Autodesk Inventor part; units mm, degrees
ref_plane "YZ Plane" through (0, 0, 0) normal (1, 0, 0) x (0, 1, 0)
ref_plane "XZ Plane" through (0, 0, 0) normal (0, 1, 0) x (-1, 0, 0)
ref_plane "XY Plane" through (0, 0, 0) normal (0, 0, 1) x (1, 0, 0)
sketch "Sketch1" plane through (0, 0, 0) normal (0, 1, 0) x (-1, 0, 0)
  line L0 (-60, 0) -> (-940, 0)
  line L1 (-891.5776, 120) -> (-60, 120)
  arc A0 (-60, 0) -> (-60, 120) centre (-60, 60) ccw
  line L2 (-60, 0) -> (-90, 0)
  arc A1 (-1909.8969, 691.9019) -> (-1970.1031, 588.0981) centre (-1940, 640) ccw
  line L3 (-1909.8969, 691.9019) -> (-951.7838, 136.1963)
  line L4 (-1970.1031, 588.0981) -> (-970.1031, 8.0981)
  arc A2 (-951.7838, 136.1963) -> (-891.5776, 120) centre (-891.5776, 240) ccw
  arc A3 (-970.1031, 8.0981) -> (-940, 0) centre (-940, 60) ccw
  line L5 (-60, 0) -> (-110, 0)
  line L6 (-110, 0) -> (-110, -100)
  line L7 (-110, -100) -> (-60, -100)
  line L8 (-60, -100) -> (-60, 0)
  line L9 (-940, 0) -> (-890, 0)
  line L10 (-890, 0) -> (-890, -100)
  line L11 (-890, -100) -> (-940, -100)
  line L12 (-940, -100) -> (-940, 0)
  line L13 (-1920.1031, 559.0981) -> (-1920.1031, -199.9999)
  line L14 (-1920.1031, -199.9999) -> (-1970.1031, -199.9999)
  line L15 (-1970.1031, -199.9999) -> (-1970.1031, 588.0981)
  point P0 (0, 0)
  dimension "d9" = 120
  dimension "d10" = 50
  dimension "d11" = 100
  dimension "d12" = 50
  dimension "d13" = 100
  dimension "d16" = 50
extrude "Extrusion1" add sketch "Sketch1" against normal blind 50 contours L8 L7 L6 L0 | L10 L11 L12 L0 | L4 L13 L14 L15
extrude "Extrusion2" add sketch "Sketch1" against normal blind 450 contours L0 A3 L4 A1 L3 A2 L1 A0
extrude "Extrusion3" add sketch "Sketch1" along normal blind 50 contours L0 A3 L4 A1 L3 A2 L1 A0
sketch "Sketch2" plane through (940, -450, 0) normal (0, 0, -1) x (-1, 0, 0)
  line L0 (880, 400) -> (880, 0)
  line L1 (880, 50) -> (830, 50)
  line L2 (830, 50) -> (830, 100)
  line L3 (830, 100) -> (880, 100)
  line L4 (880, 100) -> (880, 50)
  line L5 (0, 400) -> (0, 0)
  line L6 (0, 50) -> (50, 50)
  line L7 (50, 50) -> (50, 100)
  line L8 (50, 100) -> (0, 100)
  line L9 (0, 100) -> (0, 50)
  line L10 (-1030.1031, 50) -> (-980.1031, 50)
  line L11 (-980.1031, 50) -> (-980.1031, 100)
  line L12 (-980.1031, 100) -> (-1030.1031, 100)
  line L13 (-1030.1031, 100) -> (-1030.1031, 50)
  point P0 (940, 450)
  dimension "d24" = 50
  dimension "d25" = 50
  dimension "d26" = 50
  dimension "d27" = 50
  dimension "d28" = 50
  dimension "d29" = 50
extrude "Extrusion4" add sketch "Sketch2" along normal blind 100 contours L0 L1 L2 L3 | L8 L7 L6 L5
extrude "Extrusion5" add sketch "Sketch2" along normal blind 200 contours L13 L12 L11 L10
extrude "Extrusion6" add sketch "Sketch2" against normal blind 600 contours L13 L12 L11 L10
properties part number "FirstConveyor"
The model under review builds one solid part; all positions refer to its coordinate system, in mm. A direction names the side the tool comes from. Round coordinates to 2 decimals unless told otherwise and drop trailing zeros. Order: outer loops, then holes, each group sorted by start corner. A loop starts at its lowest first (then second) coordinate and runs counter-clockwise, first axis right, second up.
Item 1: Draft analysis for pull direction X (two halves, no side actions). For faces 4 (the flat face through (494, -204, 0)), 5 (the flat face through (1970.103, -25, 189)), 6 (the flat face through (85, -350, -49)), state which applies: released by +X, released by -X, zero draft, split by the parting line, or undercut.
Working result:
face 4: undercut
face 5: released by +X
face 6: zero draft
Item 2: Add section C-C, the plane x = 1940. State the section outline as (y, z) points.
Working result:
outline: (-450, 570.64) - (-400, 570.64) - (-400, -200) - (-350, -200) - (-350, 570.64) - (-50, 570.64) - (-50, -200) - (0, -200) - (0, 570.64) - (50, 570.64) - (50, 700) - (-450, 700) - close
Item 3: To check wall thickness, follow probe 1 along Z at (x, y) = (128, -6); probe 2 along X at (y, z) = (-392, 211.5); probe 3 along X at (y, z) = (-172, 570). State the ranges of each line that lie inside material, in increasing order.
Working result:
probe 1: z = 0 to 120
probe 2: x = 1081.62 to 1320.8, 1920.1 to 1970.1
probe 3: x = 1699.72 to 1938.9
Item 4: For pin 1 (15 mm diameter, centred on x = 927.5, z = -54.5, fed in from -Y); pin 2 (1.5 mm diameter, centred on x = 1332.5, y = -271.5, fed in from +Z); pin 3 (8 mm diameter, centred on x = 290.5, y = -17.5, fed in from -Z), all flat-tipped, find the tip position at first contact; note any pin that passes through.
Working result:
pin 1: stops at y = -400
pin 2: stops at z = 357.45
pin 3: stops at z = 0
Item 5: Add section D-D, the plane z = 60. State the section outline as (x, y) points, and give its area (3 significant figures).
Working result:
outline: (0, -450) - (1059.59, -450) - (1059.59, 50) - (0, 50) - close; (1920.1, -400) - (1970.1, -400) - (1970.1, -350) - (1920.1, -350) - close; (1920.1, -50) - (1970.1, -50) - (1970.1, 0) - (1920.1, 0) - close
area: 535,000 mm2
Item 6: Add section A-A, the plane y = -190. State the section outline as (x, z) points.
Working result:
outline: (60, 0) - (940, 0) arc R60 ccw to (970.1, 8.1) - (1970.1, 588.1) arc R60 ccw to (1909.9, 691.9) - (951.78, 136.2) arc R120 cw to (891.58, 120) - (60, 120) arc R60 ccw to start
Item 7: Machinability: for faces 1 (the flat face through (85, -50, -49)), 2 (the flat face through (890, -375, -49)), 3 (the flat face through (1945, 0, 200)), which of the approach directions +Z, -Z, +X, -X, +Y, -Y give a long, thin tool a straight path to every point of the face, cutting with its end or side? Answer none if there is none.
Working result:
face 1: -Z, +X, -X
face 2: -Z, +Y, -Y
face 3: -Z, +X, +Y
Item 8: Add section B-B, the plane z = 480. State the section outline as (x, y) points, and give its area (3 significant figures).
Working result:
outline: (1544.55, -450) - (1783.73, -450) - (1783.73, 50) - (1544.55, 50) - close; (1920.1, -400) - (1970.1, -400) - (1970.1, -350) - (1920.1, -350) - close; (1920.1, -50) - (1970.1, -50) - (1970.1, 0) - (1920.1, 0) - close
area: 125,000 mm2
